The model under review builds one solid part; all positions refer to its coordinate system, in mm. Face numbers are marked on the shaded views. Round coordinates to 2 decimals unless told otherwise and drop trailing zeros. Order: outer loops, then holes, each group sorted by start corner. A loop starts at its lowest first (then second) coordinate and runs counter-clockwise, first axis right, second up. Notation, with made-up numbers: (6, -10.75) -> (62, -10.75) arc R27 cw to (62, 13.25) -> close; hole circle Ø2 at (46.5, -22). An arc over 180 degrees is marked (long way). Put each result on its own line as item: value. Start each with the question number.
from build123d import *

# Parameters (mm, degrees)
F0_R     = 25.4
F1_DEPTH = 24.3078
F1_TAPER = 45
F3_W     = 50.8
F3_H     = 26.1644069105
F4_DEPTH = 28.448
F2_R     = 22.225
F5_DEPTH = 18.034
F5_TAPER = 45


with BuildPart() as f1:
    # F0 (on Front) → F1 (new body)
    with BuildSketch(Plane.XZ):
        Circle(F0_R)
    extrude(amount=F1_DEPTH, taper=F1_TAPER)

    # F3 (on face) → F4 (cut)
    with BuildSketch(Plane(origin=(0, 0, 0), x_dir=(-1, 0, 0), z_dir=(0, 1, 0))):
        with Locations((0, -13.0822034553)):
            Rectangle(F3_W, F3_H)
    extrude(amount=-F4_DEPTH, mode=Mode.SUBTRACT)

    # F2 (on face) → F5 (cut)
    with BuildSketch(Plane(origin=(0, 0, 0), x_dir=(-1, 0, 0), z_dir=(0, 1, 0))):
        Circle(F2_R)
    extrude(amount=-F5_DEPTH, taper=F5_TAPER, mode=Mode.SUBTRACT)


solid = f1.part
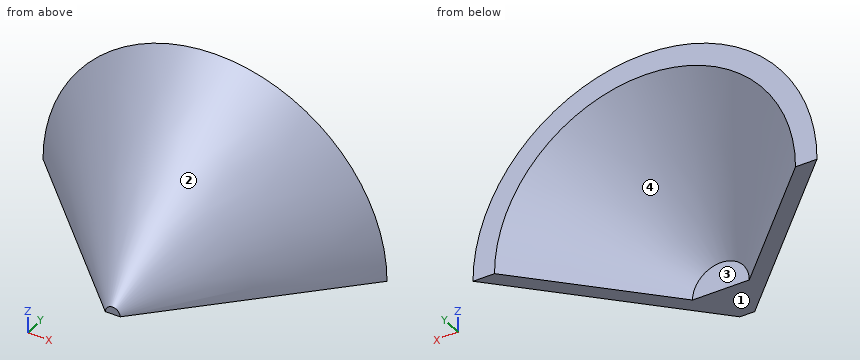
Q1. Take a section at A-A on x = 0. Give the boundary of the cut face in (y, z) (3 decimals).
Q2. Take a section at C-C on y = -14.25. Give the boundary of the cut face in (x, z) (3 decimals), and give its area (3 significant figures).
Q3. Wall thickness on probe 1 along X at (y, z) = (-3.25, 13); probe 2 along X at (y, z) = (-2.5, 13.75); probe 3 along Y at (x, z) = (-15.5, 12.25): over which ranges is each line inside the solid? List them lowest first. Write a range as [from, to].
Q4. Clearance check with flat-ended pins moving along their axes: pin 1 Ø6 at (x, z) = (8, 10.5) entering from +Y; pin 2 Ø5 at (y, z) = (-4.5, 8.5) entering from +X; pin 3 Ø6 at (y, z) = (-9.5, 13) entering from +X. State where each tip first meets the part, or that it passes through.
Q5. Draft analysis for pull direction X (two halves, no side actions). For the marked faces 1, 2, 3 and 4, state which applies: +X half, -X half, draft (parallel to the pull), parting line (faces both ways), or undercut.
Q6. Take a section at B-B on y = -10.5. Give the boundary of the cut face in (x, z) (3 decimals), and give its area (3 significant figures).
Calculated:
1. outline: (-24.308, 0) -> (-18.034, 0) -> (-18.034, 4.191) -> (0, 22.225) -> (0, 25.4) -> (-24.308, 1.092) -> close
2. outline: (-11.15, 0) -> (-7.975, 0) arc R7.975 cw to (7.975, 0) -> (11.15, 0) arc R11.15 ccw to start
2. area: 95.4 mm²
3. probe 1: x = [-17.93, -13.82], [13.82, 17.93]
3. probe 2: x = [-18.31, -14.14], [14.14, 18.31]
3. probe 3: y = [-5.64, -2.47]
4. pin 1: stops at y = -6.02
4. pin 2: stops at x = 21.96
4. pin 3: stops at x = 14.49
5. face 1: draft
5. face 2: parting line
5. face 3: undercut
5. face 4: undercut
6. outline: (-14.9, 0) -> (-11.725, 0) arc R11.725 cw to (11.725, 0) -> (14.9, 0) arc R14.9 ccw to start
6. area: 133 mm²
